Input: part model. Units: mm. Frame: model coordinates. Round coordinates to 2 decimals unless told otherwise and drop trailing zeros. Order: outer loops, then holes, each group sorted by start corner. A loop starts at its lowest first (then second) coordinate and runs counter-clockwise, first axis right, second up. Notation, with made-up numbers: (-25.75, -26) - (8.25, -26) arc R17 ccw to (8.25, -2) - close; hole circle Ø4 at (-34.75, 40.25). An arc over 180 degrees is marked (long way). One line per item, written item: value. Start each with the question number.
from build123d import *

# Parameters (mm, degrees)
F0_R     = 10
F1_DEPTH = 1915
F2_R     = 7.5
F3_DEPTH = 55
F4_R     = 7.5
F5_DEPTH = 10
F8_DEPTH = 2
F9_SIZE  = 1


with BuildPart() as f1:
    # F0 (on Front) → F1 (new body)
    with BuildSketch(Plane.XZ):
        Circle(F0_R)
    extrude(amount=F1_DEPTH)

    # F2 (on face) → F3 (join)
    with BuildSketch(Plane.XZ.offset(1915)):
        Circle(F2_R)
    extrude(amount=F3_DEPTH)

    # F4 (on face) → F5 (join)
    with BuildSketch(Plane(origin=(0, 0, 0), x_dir=(-1, 0, 0), z_dir=(0, 1, 0))):
        Circle(F4_R)
    extrude(amount=F5_DEPTH)

    # F7 (on offset) → F8 (cut)
    with BuildSketch(Plane.XY.offset(7.5)):
        with BuildLine():
            Line((1.997144, -1965.893146), (1.997144, -1960.106854))
            ThreePointArc((1.997144, -1960.106854), (0.000708, -1958), (-1.997219, -1960.105441))
            Line((-1.997219, -1960.105441), (-1.997219, -1965.894559))
            Line((-1.997219, -1965.894559), (-1.997219, -1966.105441))
            ThreePointArc((-1.997219, -1966.105441), (-0.000708, -1968), (1.997144, -1966.106854))
            Line((1.997144, -1966.106854), (1.997144, -1965.893146))
        make_face()
        with BuildLine():
            ThreePointArc((1.997144, -1966.106854), (2, -1966), (1.997144, -1965.893146))
            Line((1.997144, -1965.893146), (1.997144, -1966.106854))
        make_face()
        with BuildLine():
            Line((-1.997219, -1966.105441), (-1.997219, -1965.894559))
            ThreePointArc((-1.997219, -1965.894559), (-2, -1966), (-1.997219, -1966.105441))
        make_face()
    extrude(amount=-F8_DEPTH, mode=Mode.SUBTRACT)

    # F9
    f9_edges = [f1.edges().sort_by_distance(p)[0] for p in [
        (-7.5, -1970, 0),
        (7.5, 10, 0),
    ]]
    chamfer(f9_edges, length=F9_SIZE)


solid = f1.part
Item 1: First-contact query: pin 1 Ø1.4 at (y, z) = (-1964, 6) entering from +X; pin 2 Ø4 at (y, z) = (-301, 3) entering from -X; pin 3 Ø1.2 at (x, y) = (0, -1963) entering from +Z. Flat tips, straight axial feed; report the tip coordinate or a pass-through.
Item 2: Line query: L1, parallel to Y at x = 8, z = 1.5; L2, parallel to Z at x = -2.5, y = -1764; L3, parallel to Z at x = -6.75, y = -307. Output: solid intervals per line, ascending.
Item 3: Section query A-A on y = -942. Return loops of the section in (x, z).
Geometry results:
1. pin 1: stops at x = 5.31
1. pin 2: stops at x = -9.95
1. pin 3: stops at z = 5.5
2. L1: y = -1915 to 0
2. L2: z = -9.68 to 9.68
2. L3: z = -7.38 to 7.38
3. outline: circle Ø20 at (0, 0)
